from build123d import *

# Parameters (mm, degrees)
F0_W     = 60
F0_H     = 79
F0_R     = 1.5
F1_DEPTH = 3
F2_W     = 34
F2_H     = 58
F3_DEPTH = 3
F4_R     = 5
F5_R     = 5


with BuildPart() as f1:
    # F0 (on Top) → F1 (new body)
    with BuildSketch(Plane.XY):
        Rectangle(F0_W, F0_H)
        with Locations((-24, -23.5)):
            Circle(F0_R, mode=Mode.SUBTRACT)
        with Locations((24, -23.5)):
            Circle(F0_R, mode=Mode.SUBTRACT)
        with Locations((-24, 34.5)):
            Circle(F0_R, mode=Mode.SUBTRACT)
        with Locations((24, 34.5)):
            Circle(F0_R, mode=Mode.SUBTRACT)
    extrude(amount=F1_DEPTH)

    # F2 (on face) → F3 (cut, through all)
    with BuildSketch(Plane.XY.offset(3)):
        Rectangle(F2_W, F2_H)
    extrude(amount=-F3_DEPTH, mode=Mode.SUBTRACT)

    # F4
    f4_edges = [f1.edges().sort_by_distance(p)[0] for p in [
        (-17, 29, 1.5),
    ]]
    fillet(f4_edges, radius=F4_R)

    # F5
    f5_edges = [f1.edges().sort_by_distance(p)[0] for p in [
        (-17, -29, 1.5),
        (17, -29, 1.5),
        (17, 29, 1.5),
    ]]
    fillet(f5_edges, radius=F5_R)


solid = f1.part
Can you work these out from the model? Positions are in its coordinate system, mm. A direction names the side the tool comes from. Coordinates: 2 decimals unless noted, no trailing zeros. Loops run counter-clockwise (first coordinate to the right, second up) from the corner with the lowest first, then second, coordinate; pieces in that order, holes last. Notation, with made-up numbers: (7.5, 50.5) - (54.5, 50.5) arc R23 cw to (54.5, 86.5) - close; hole circle Ø1 at (64, -10). An arc over 180 degrees is marked (long way). Answer as a JSON object with one key per item and string values. Group by question number.
Item 1: If we section it at C-C (y = 34.5): List the corners of the cut face in (x, z) for me, plus the area to 3 significant figures.
Item 2: If we mould it in two halves opening along X, with no side actions, what happens to faces 1 (the face through (-15, 28, 1)), 2 (the face through (0, 39.5, 1)), 3 (the face through (30, -1, 1))? For each: released by +X, released by -X, zero draft, split by the parting line, or undercut.
Item 3: If I drill on L1, parallel to Y at x = 24, z = 1.3; L2, parallel to Y at x = -1, z = 2.6; L3, parallel to X at y = -21, z = 2.35, over which ranges is the centre line in solid material (lowest first)? Write a range as from..to.
Item 4: If we section it at A-A (x = 24): List the corners of the cut face in (y, z) for me.
Item 5: If we section it at B-B (z = 1.95): List the corners of the cut face in (x, y) for me, plus the area to 3 significant figures.
Item 6: If we section it at D-D (y = -5.5): List the corners of the cut face in (x, z) for me.
Item 7: On a 3-axis mill with a long thin cutter (end or side, diameter ignored), from which of +Z, -Z, +X, -X, +Y, -Y can I reach the whole of each face in a straight line? I mean faces 4 (the face through (0, -39.5, 1)), 5 (the face through (0, -29, 2)). Say none if no direction works.
Returned:
{
 "1": {"outline": "(-30, 0) - (-25.5, 0) - (-25.5, 3) - (-30, 3) - close; (-22.5, 0) - (22.5, 0) - (22.5, 3) - (-22.5, 3) - close; (25.5, 0) - (30, 0) - (30, 3) - (25.5, 3) - close", "area": "162 mm²"},
 "2": {"face 1": "undercut", "face 2": "zero draft", "face 3": "released by +X"},
 "3": {"L1": "y = -39.5..-25, -22..33, 36..39.5", "L2": "y = -39.5..-29, 29..39.5", "L3": "x = -30..-17, 17..30"},
 "4": {"outline": "(-39.5, 0) - (-25, 0) - (-25, 3) - (-39.5, 3) - close; (-22, 0) - (33, 0) - (33, 3) - (-22, 3) - close; (36, 0) - (39.5, 0) - (39.5, 3) - (36, 3) - close"},
 "5": {"outline": "(-30, -39.5) - (30, -39.5) - (30, 39.5) - (-30, 39.5) - close; hole circle Ø3 at (-24, -23.5); hole circle Ø3 at (-24, 34.5); hole (-17, -24) arc R5 ccw to (-12, -29) - (12, -29) arc R5 ccw to (17, -24) - (17, 24) arc R5 ccw to (12, 29) - (-12, 29) arc R5 ccw to (-17, 24) - close; hole circle Ø3 at (24, -23.5); hole circle Ø3 at (24, 34.5)", "area": "2,760 mm²"},
 "6": {"outline": "(-30, 0) - (-17, 0) - (-17, 3) - (-30, 3) - close; (17, 0) - (30, 0) - (30, 3) - (17, 3) - close"},
 "7": {"face 4": "+Z, -Z, +X, -X, -Y", "face 5": "+Z, -Z"}
}
